Input: dimensioned drawing with shaded views. Units: mm. Origin: part minimum x, y, z. A direction names the side the tool comes from. Coordinates: 2 decimals unless noted, no trailing zeros. Order: outer loops, then holes, each group sorted by start corner. A loop starts at its lowest first (then second) coordinate and runs counter-clockwise, first axis right, second up. Notation, with made-up numbers: (7, -27) - (27, -27) arc R9 ccw to (27, -10) - close; hole circle Ø9 at (86.5, 71.25). An arc over 180 degrees is marked (long way). One line per question, with ' | ' between items. Start each with the question number.
(1) Section A-A (x = 12.05). Return the cut outline in (y, z).
(2) Section C-C (z = 7.25). Return the cut outline in (x, y), then the cut area to 3 significant figures.
(3) Draft query along Y for the marked faces 3, 4 and 5. Return one class per face: +Y half, -Y half, draft (parallel to the pull), parting line (faces both ways), or undercut.
(4) Line query: line 1 along X through (y, z) = (12.25, 6.5); line 2 along Y through (x, z) = (12.05, 5.15); line 3 along Z through (x, y) = (7.25, 17.75). Output: solid intervals per line, ascending.
(5) Contact query for flat-ended pins moving along their axis: P1, Ø2, axis at x = 13.5, z = 2, coming from the +Y side; P2, Ø8, axis at x = 12, y = 15.5, coming from the +Z side; P3, Ø6, axis at y = 20, z = 8.5, coming from the -X side. Output: stop coordinate, or through.
(6) Section D-D (z = 9.5). Return the cut outline in (x, y).
(7) Access query for the marked faces 1 and 2. Directions: +Z, -Z, +X, -X, +Y, -Y. A direction counts if a zero-diameter tool reaches every point of the face in a straight line with its end or side. Return the directions, or none.
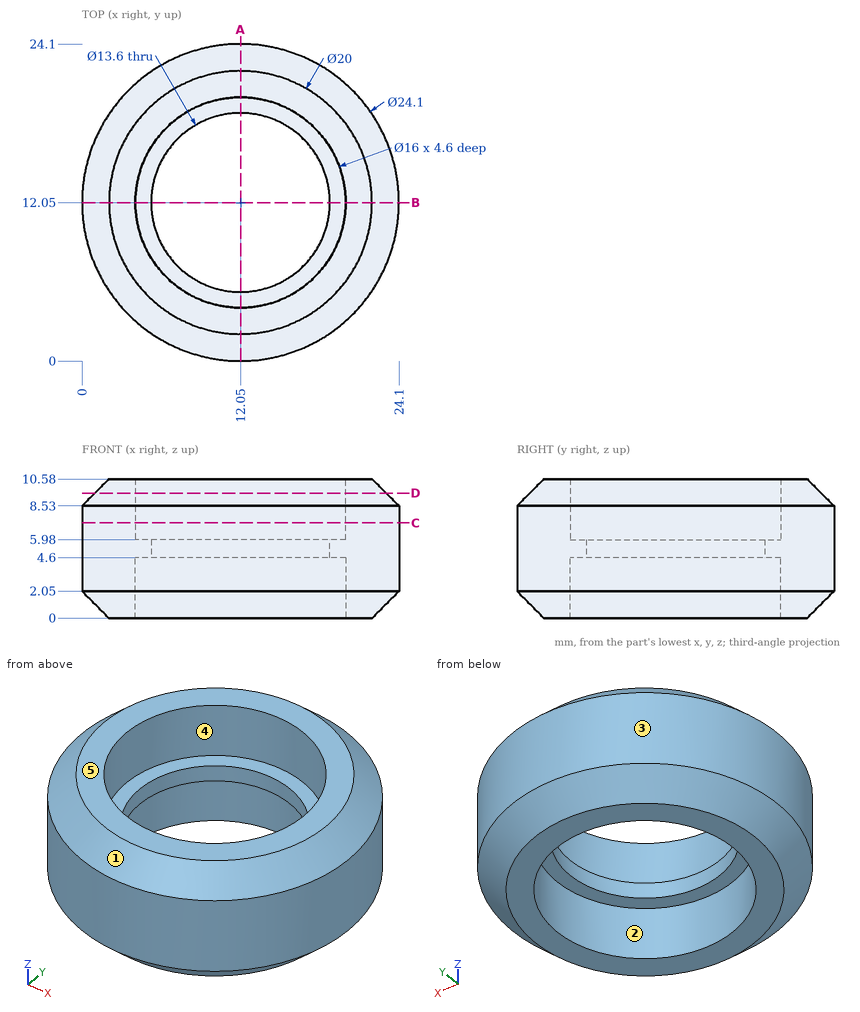
Response values:
1) outline: (0, 2.05) - (2.05, 0) - (4.05, 0) - (4.05, 4.6) - (5.25, 4.6) - (5.25, 5.98) - (4.05, 5.98) - (4.05, 10.58) - (2.05, 10.58) - (0, 8.53) - close; (18.85, 4.6) - (20.05, 4.6) - (20.05, 0) - (22.05, 0) - (24.1, 2.05) - (24.1, 8.53) - (22.05, 10.58) - (20.05, 10.58) - (20.05, 5.98) - (18.85, 5.98) - close
2) outline: circle Ø24.1 at (12.05, 12.05); hole circle Ø16 at (12.05, 12.05) | area: 255 mm²
3) face 3: parting line | face 4: undercut | face 5: draft
4) line 1: x = 0 to 4.05, 20.05 to 24.1 | line 2: y = 0 to 5.25, 18.85 to 24.1 | line 3: z = 4.6 to 5.98
5) P1: stops at y = 24.09 | P2: stops at z = 5.98 | P3: stops at x = 1.06
6) outline: circle Ø22.16 at (12.05, 12.05); hole circle Ø16 at (12.05, 12.05)
7) face 1: +Z | face 2: -Z
